Work out the finished part from the listing and answer in its coordinate system (mm). Face numbers are marked on the shaded views. A direction names the side the tool comes from. Coordinates: 2 decimals unless noted, no trailing zeros. Loops run counter-clockwise (first coordinate to the right, second up) from the corner with the lowest first, then second, coordinate; pieces in that order, holes last. Notation, with made-up numbers: (21, -6) -> (38, -6) arc R12 cw to (38, 14) -> close; hole circle Ø11 at (-31, 84.5). An arc over 180 degrees is marked (long way). Use a Markdown table: item, result.
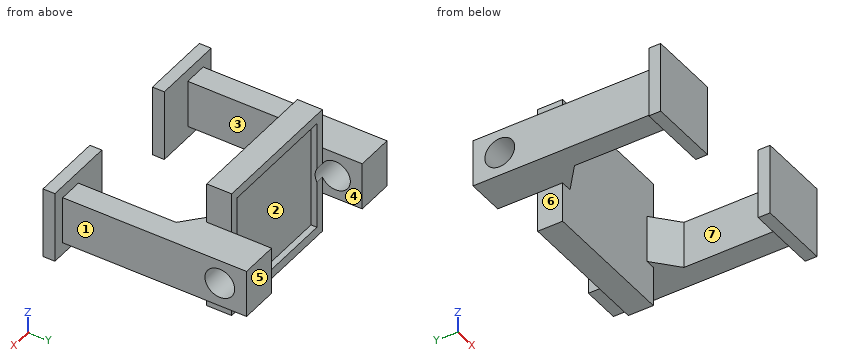
from build123d import *

# Parameters (mm, degrees)
SKETCH1_W            = 14.732
SKETCH1_H            = 13.716
BOSS_EXTRUDE1_DEPTH  = 2.032
SKETCH6_W            = 25.4
SKETCH6_H            = 5.08
BOSS_EXTRUDE2_DEPTH  = 12.7
SKETCH16_W           = 7.62
SKETCH16_H           = 7.62
BOSS_EXTRUDE5_DEPTH  = 1.27
SKETCH15_W           = 1.27
SKETCH15_H           = 12.7
SKETCH15_W_2         = 1.31
CUT_EXTRUDE5_DEPTH   = 10
SKETCH17_W           = 4.024
SKETCH17_H           = 5.08
BOSS_EXTRUDE10_DEPTH = 6.9215
SKETCH21_W           = 4.064
SKETCH21_H           = 5.08
BOSS_EXTRUDE11_DEPTH = 6.9215
SKETCH24_W           = 14.732
SKETCH24_H           = 13.716
SKETCH24_W_2         = 12.954
SKETCH24_H_2         = 11.684
BOSS_EXTRUDE12_DEPTH = 0.635
SKETCH23_R           = 1.5875
CUT_EXTRUDE6_DEPTH   = 25.7175


with BuildPart() as part:
    # Sketch1 → Boss-Extrude1 (new body)
    with BuildSketch(Plane(origin=(0, 0, 0), x_dir=(1, 0, 0), z_dir=(0, 1, 0))):
        Rectangle(SKETCH1_W, SKETCH1_H)
    extrude(amount=BOSS_EXTRUDE1_DEPTH)

    # Sketch6 → Boss-Extrude2 (add)
    with BuildSketch(Plane(origin=(0, 0, 0), x_dir=(-1, 0, 0), z_dir=(0, -1, 0))):
        Rectangle(SKETCH6_W, SKETCH6_H)
    extrude(amount=BOSS_EXTRUDE2_DEPTH)

    # Sketch16 → Boss-Extrude5 (add)
    with BuildSketch(Plane.XZ.offset(12.7)):
        with Locations((8.89, 0)):
            Rectangle(SKETCH16_W, SKETCH16_H)
        with Locations((-8.89, 0)):
            Rectangle(SKETCH16_W, SKETCH16_H)
    extrude(amount=BOSS_EXTRUDE5_DEPTH)

    # Sketch15 → Cut-Extrude5 (cut)
    with BuildSketch(Plane(origin=(0, 0, -2.54), x_dir=(-1, 0, 0), z_dir=(0, 0, -1))):
        with Locations((-12.065, -6.35)):
            Rectangle(SKETCH15_W, SKETCH15_H)
        Polygon((-8.89, -2.27), (-8.89, -12.7), (8.89, -12.7), (8.89, -2.27), (6.166, 0), (-6.35, 0), align=None)
        with Locations((12.045, -6.35)):
            Rectangle(SKETCH15_W_2, SKETCH15_H)
    extrude(amount=-CUT_EXTRUDE5_DEPTH, mode=Mode.SUBTRACT)

    # Sketch17 → Boss-Extrude10 (add)
    with BuildSketch(Plane(origin=(0, 0, 0), x_dir=(1, 0, 0), z_dir=(0, 1, 0))):
        with Locations((-9.378, 0)):
            Rectangle(SKETCH17_W, SKETCH17_H)
    extrude(amount=BOSS_EXTRUDE10_DEPTH)

    # Sketch21 → Boss-Extrude11 (add)
    with BuildSketch(Plane(origin=(0, 0, 0), x_dir=(1, 0, 0), z_dir=(0, 1, 0))):
        with Locations((9.398, 0)):
            Rectangle(SKETCH21_W, SKETCH21_H)
    extrude(amount=BOSS_EXTRUDE11_DEPTH)

    # Sketch24 → Boss-Extrude12 (add)
    with BuildSketch(Plane(origin=(0, 2.032, 0), x_dir=(1, 0, 0), z_dir=(0, 1, 0))):
        Rectangle(SKETCH24_W, SKETCH24_H)
        Rectangle(SKETCH24_W_2, SKETCH24_H_2, mode=Mode.SUBTRACT)
    extrude(amount=BOSS_EXTRUDE12_DEPTH)

    # Sketch23 → Cut-Extrude6 (cut)
    with BuildSketch(Plane.ZY.offset(11.39)):
        with Locations((0, 4.064)):
            Circle(SKETCH23_R)
    extrude(amount=-CUT_EXTRUDE6_DEPTH, mode=Mode.SUBTRACT)


solid = part.part
Q1. Section C-C on x = 8 is taken. Determine the outline of the cut face in (y, z) (1 decimal), and give its area (3 significant figures).
Solved:
| item | result |
|---|---|
| outline | (-14, -3.8) -> (-12.7, -3.8) -> (-12.7, 3.8) -> (-14, 3.8) -> close; (-1.5, -2.5) -> (6.9, -2.5) -> (6.9, 2.5) -> (-1.5, 2.5) -> close; hole circle Ø3.2 at (4.1, 0) |
| area | 44.4 mm² |
Q2. For the marked faces 1, 2, 3 and 4, determine the directions among +Z, -Z, +X, -X, +Y, -Y from which every point of the face is accessible in a straight line to the end or side of a thin tool.
Solved:
| item | result |
|---|---|
| face 1 | +Z, -Z, +X, +Y |
| face 2 | +Y |
| face 3 | +Z, -Z |
| face 4 | +Z, -Z, +Y |
Q3. Determine the mould class of the marked faces 5, 6 and 7 for opening direction Y: pulls with the +Y half, pulls with the -Y half, needs draft (parallel to the pull), parting line crosses it, or undercut.
Solved:
| item | result |
|---|---|
| face 5 | pulls with the +Y half |
| face 6 | needs draft |
| face 7 | undercut |
Q4. Given pin 1 Ø5 at (x, z) = (0.5, -1.5) entering from +Y; pin 2 Ø8 at (y, z) = (-7, 3.5) entering from +X; pin 3 Ø4 at (x, z) = (1.5, -2.5) entering from -Y; pin 4 Ø1.5 at (x, y) = (-1, 4.5) entering from -Z, each flat-ended and moving along its own axis, determine where each tip first touches the part or whether it passes through.
Solved:
| item | result |
|---|---|
| pin 1 | y = 2.03 |
| pin 2 | x = 11.43 |
| pin 3 | y = 0 |
| pin 4 | through |
Q5. Section A-A on z = -3.5 is taken. Determine the outline of the cut face in (x, y).
Solved:
| item | result |
|---|---|
| outline | (-12.7, -13.97) -> (-5.08, -13.97) -> (-5.08, -12.7) -> (-12.7, -12.7) -> close; (-7.37, 0) -> (7.37, 0) -> (7.37, 2.67) -> (6.48, 2.67) -> (6.48, 2.03) -> (-6.48, 2.03) -> (-6.48, 2.67) -> (-7.37, 2.67) -> close; (5.08, -13.97) -> (12.7, -13.97) -> (12.7, -12.7) -> (5.08, -12.7) -> close |
Q6. Section D-D on x = -4.25 is taken. Determine the outline of the cut face in (y, z).
Solved:
| item | result |
|---|---|
| outline | (0, -6.86) -> (2.67, -6.86) -> (2.67, -5.84) -> (2.03, -5.84) -> (2.03, 5.84) -> (2.67, 5.84) -> (2.67, 6.86) -> (0, 6.86) -> close |
Q7. Consider line 1 (X direction, y = -4, z = 2); line 2 (Y direction, x = 10, z = 0); line 3 (Y direction, x = -5.75, z = -3.5). Determine where each line is inside the solid, lowest interval first. Write a range as [from, to].
Solved:
| item | result |
|---|---|
| line 1 | [-11.39, -8.89], [8.89, 11.43] |
| line 2 | [-13.97, 2.48], [5.65, 6.92] |
| line 3 | [-13.97, -12.7], [0, 2.03] |
Q8. Section B-B on y = -3 is taken. Determine the outline of the cut face in (x, z), and give its area (3 significant figures).
Solved:
| item | result |
|---|---|
| outline | (-11.39, -2.54) -> (-8.89, -2.54) -> (-8.89, 2.54) -> (-11.39, 2.54) -> close; (8.89, -2.54) -> (11.43, -2.54) -> (11.43, 2.54) -> (8.89, 2.54) -> close |
| area | 25.6 mm² |
